Geometry: final body of the model. Coordinates: model frame, mm. Give positions to 0.01 mm unless a question says otherwise; leave off trailing zeros. Loops run counter-clockwise (first coordinate to the right, second up) from the corner with the lowest first, then second, coordinate; pieces in that order, holes last.
from build123d import *

# Parameters (mm, degrees)
SKETCH1_R           = 9.525
SKETCH1_R_2         = 8.636
BOSS_EXTRUDE1_DEPTH = 609.6
SKETCH3_R           = 20.246819027
CUT_EXTRUDE1_DEPTH  = 101.6


with BuildPart() as part:
    # Sketch1 → Boss-Extrude1 (new body)
    with BuildSketch(Plane.XY):
        Circle(SKETCH1_R)
        Circle(SKETCH1_R_2, mode=Mode.SUBTRACT)
    extrude(amount=BOSS_EXTRUDE1_DEPTH)

    # Sketch2 → Revolve1 (revolve)
    with BuildSketch(Plane(origin=(0, 0, 0), x_dir=(0, 0, -1), z_dir=(1, 0, 0))):
        with BuildLine():
            Line((-61.9125, 9.525), (0, 9.525))
            Line((0, 9.525), (0, 17.78))
            Line((0, 17.78), (-25.722714052, 17.78))
            ThreePointArc((-25.722714052, 17.78), (-24.855324241, 16.552662429), (-24.549271858, 15.08125))
            ThreePointArc((-24.549271858, 15.08125), (-29.710775793, 11.697210877), (-30.756012676, 17.78))
            Line((-30.756012676, 17.78), (-46.83125, 17.78))
            Line((-46.83125, 17.78), (-46.83125, 12.7))
            Line((-46.83125, 12.7), (-61.9125, 12.7))
            Line((-61.9125, 12.7), (-61.9125, 9.525))
        make_face()
    revolve(axis=Axis((0, 0, 0), (0, 0, 1)))

    # Sketch3 → Cut-Extrude1 (cut)
    with BuildSketch(Plane(origin=(0, 0, 0), x_dir=(-1, 0, 0), z_dir=(0, 0, -1))):
        Circle(SKETCH3_R)
        Polygon((14.664696837, 0), (7.332348419, 12.7), (-7.332348419, 12.7), (-14.664696837, 0), (-7.332348419, -12.7), (7.332348419, -12.7), align=None, mode=Mode.SUBTRACT)
    extrude(amount=-CUT_EXTRUDE1_DEPTH, mode=Mode.SUBTRACT)


solid = part.part
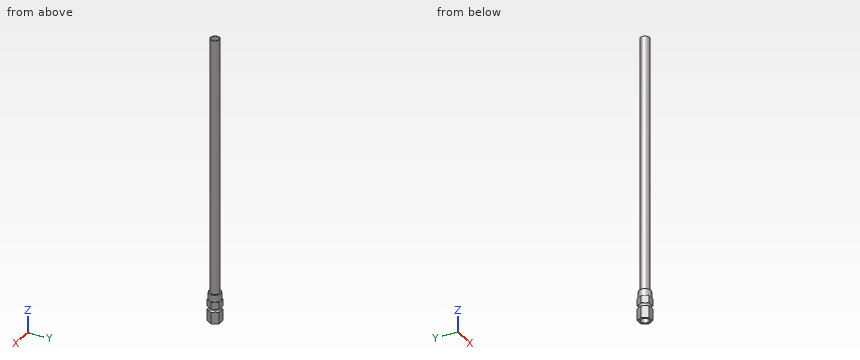
Item 1: Section query A-A on z = 543.5. Return loops of the section in (x, y) (3 decimals), plus the area to 3 significant figures.
Values follow:
outline: circle Ø19.05 at (0, 0); hole circle Ø17.272 at (0, 0)
area: 50.7 mm2
Item 2: Pin query (flat end, axial travel): pin 1 (7 mm diameter, centred on x = -3.5, y = 10.5, fed in from +Z); pin 2 (8 mm diameter, centred on y = -6.5, z = 497.5, fed in from -X); pin 3 (14 mm diameter, centred on x = 0, y = 0, fed in from +Z); pin 4 (8 mm diameter, centred on y = -4.5, z = 284, fed in from -X). Return the tip coordinate at first contact, or that it passes through.
Values follow:
pin 1: stops at z = 609.6
pin 2: stops at x = -9.19
pin 3: passes through
pin 4: stops at x = -9.51
Item 3: Ray query, probe 1 along Y at (x, z) = (0, 420) (3 decimals); probe 2 along X at (y, z) = (0.75, 185.5); probe 3 along Z at (x, y) = (-10, -5). Return the intervals inside material, ascending.
Values follow:
probe 1: y = -9.525 to -8.636, 8.636 to 9.525
probe 2: x = -9.5 to -8.6, 8.6 to 9.5
probe 3: z = 0 to 61.91
